Design review of the part built by this model. Coordinates are the model's own, in mm. A direction names the side the tool comes from. Coordinates: 2 decimals unless noted, no trailing zeros. Write each loop counter-clockwise with the first axis right and the second up, starting at its lowest first coordinate (ties: lowest second). Pieces come first, ordered by that corner, then holes. Notation, with made-up numbers: (2.5, 61) -> (18.5, 61) arc R31 cw to (18.5, 92) -> close; hole circle Ø10 at (58.25, -39.75). An arc over 180 degrees is marked (long way). Answer in a Markdown table with one row per item. Add a question column.
Item 1: For faces 4 (the face through (0, 2, 12.738)), 5 (the face through (-1, 4.6, 0)), list the 3-axis set-ups (+Z, -Z, +X, -X, +Y, -Y) from which the entire face can be reached by the end or side of a thin tool; tool diameter is ignored.
Item 2: Draft analysis for pull direction X (two halves, no side actions). For faces 1 (the face through (-1, 2, -28)), 2 (the face through (40, 2, 0)), 3 (the face through (34.313, 2.268, -20.068)), state which applies: released by +X, released by -X, zero draft, split by the parting line, or undercut.
Item 3: Take a section at B-B, the plane x = 31.75. Write out the cut boundary in (y, z), and give its area (3 significant figures).
Item 4: Take a section at D-D, the plane z = -22. Write out the cut boundary in (x, y), and give its area (3 significant figures).
Item 5: To check wall thickness, follow line 1 (Z direction, x = 6.5, y = 0.55); line 2 (Z direction, x = -31.75, y = 3.65); line 3 (X direction, y = 2.55, z = 21). State the ranges of each line that lie inside material, in increasing order.
Item 6: Take a section at A-A, the plane z = 9. Write out the cut boundary in (x, y), and give its area (3 significant figures).
Item 7: Clearance check with a flat-ended pin moving along its axis: P1, Ø4.5, axis at x = -31.75, z = 20.64, coming from the +Y side. State where the tip first meets the part, or that it passes through.
Item 8: Take a section at C-C, the plane y = 2.85. Give the number of separate pieces and of enclosed holes in the cut face, and give its area (3 significant figures).
from build123d import *

# Parameters (mm, degrees)
SKETCH_3_W          = 80
SKETCH_3_H          = 56
EXTRUDE_1_DEPTH     = 4.6
SKETCH_1_R          = 2.625
SKETCH_1_W          = 40.4
SKETCH_1_H          = 4.6
CUT_EXTRUDE_1_DEPTH = 4.6
FILLET_2_R          = 4


with BuildPart() as part:
    # 草图3 → 凸台-拉伸1 (new body)
    with BuildSketch(Plane(origin=(0, 0, 0), x_dir=(1, 0, 0), z_dir=(0, 1, 0))):
        Rectangle(SKETCH_3_W, SKETCH_3_H)
    extrude(amount=EXTRUDE_1_DEPTH)

    # 草图1 → 切除-拉伸1 (cut)
    with BuildSketch(Plane(origin=(0, 0, 0), x_dir=(1, 0, 0), z_dir=(0, 1, 0))):
        with Locations(Location((-31.75, 20.6375, 0), (0, 0, 90))):
            Circle(SKETCH_1_R)
        with Locations(Location((31.75, 20.6375, 0), (0, 0, 90))):
            Circle(SKETCH_1_R)
        with Locations(Location((31.75, -20.6375, 0), (0, 0, 90))):
            Circle(SKETCH_1_R)
        with Locations(Location((-31.75, -20.6375, 0), (0, 0, 90))):
            Circle(SKETCH_1_R)
        with Locations((0, -10.4375)):
            Rectangle(SKETCH_1_W, SKETCH_1_H)
        with Locations((0, 10.4375)):
            Rectangle(SKETCH_1_W, SKETCH_1_H)
    extrude(amount=CUT_EXTRUDE_1_DEPTH, mode=Mode.SUBTRACT)

    # 圆角2
    fillet_2_edges = [part.edges().sort_by_distance(p)[0] for p in [
        (40, 2.3, 28),
        (-40, 2.3, 28),
        (-40, 2.3, -28),
        (40, 2.3, -28),
    ]]
    fillet(fillet_2_edges, radius=FILLET_2_R)


solid = part.part
Answers:
| question | item | result |
|---|---|---|
| 1 | face 4 | +Y, -Y |
| 1 | face 5 | +Z, -Z, +X, -X, +Y |
| 2 | face 1 | zero draft |
| 2 | face 2 | released by +X |
| 2 | face 3 | undercut |
| 3 | outline | (0, -28) -> (4.6, -28) -> (4.6, -23.26) -> (0, -23.26) -> close; (0, -18.01) -> (4.6, -18.01) -> (4.6, 18.01) -> (0, 18.01) -> close; (0, 23.26) -> (4.6, 23.26) -> (4.6, 28) -> (0, 28) -> close |
| 3 | area | 209 mm^2 |
| 4 | outline | (-40, 0) -> (-33.99, 0) -> (-33.99, 4.6) -> (-40, 4.6) -> close; (-29.51, 0) -> (29.51, 0) -> (29.51, 4.6) -> (-29.51, 4.6) -> close; (33.99, 0) -> (40, 0) -> (40, 4.6) -> (33.99, 4.6) -> close |
| 4 | area | 327 mm^2 |
| 5 | line 1 | z = -28 to -12.74, -8.14 to 8.14, 12.74 to 28 |
| 5 | line 2 | z = -28 to -23.26, -18.01 to 18.01, 23.26 to 28 |
| 5 | line 3 | x = -40 to -34.35, -29.15 to 29.15, 34.35 to 40 |
| 6 | outline | (-40, 0) -> (-20.2, 0) -> (-20.2, 4.6) -> (-40, 4.6) -> close; (20.2, 0) -> (40, 0) -> (40, 4.6) -> (20.2, 4.6) -> close |
| 6 | area | 182 mm^2 |
| 7 | P1 | passes through |
| 8 | separate pieces | 1 |
| 8 | enclosed holes | 6 |
| 8 | area | 4,010 mm^2 |
